For this review, use the dimensioned drawing (mm, ordinates from the lowest corner) and the shaded views. Round coordinates to 2 decimals unless told otherwise and drop trailing zeros. Write each loop counter-clockwise with the first axis right and the second up, starting at its lowest first coordinate (ties: lowest second). Pieces come first, ordered by that corner, then holes. Notation, with made-up numbers: M -28,81 L -7,81 A31 ccw -7,119 Z; hole C 64.5,-10.75 d8. An arc over 180 degrees is marked long. Answer in a Markdown table with one row per item.
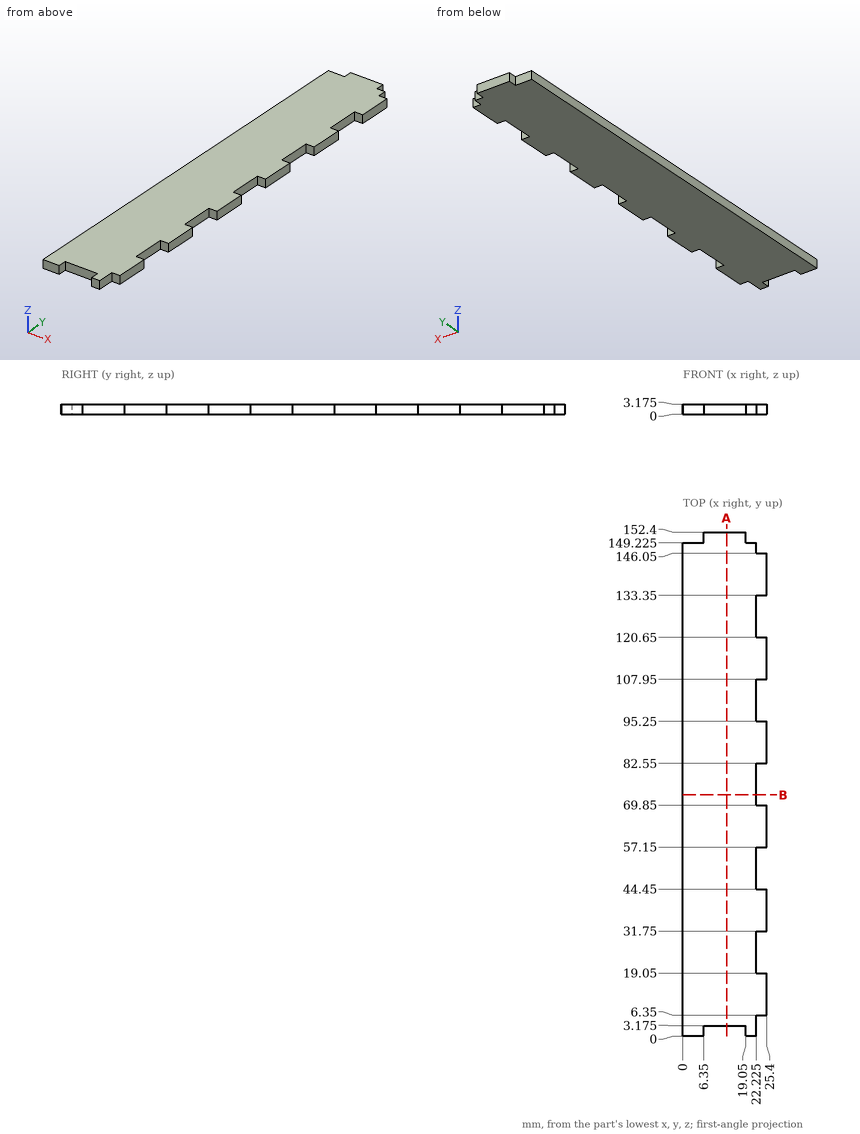
Q1. Take a section at B-B (y = 73). State the section outline as (x, z) points (3 decimals).
Found:
| item | result |
|---|---|
| outline | M 0,0 L 22.225,0 L 22.225,3.175 L 0,3.175 Z |
Q2. Insertion check: P1, Ø1.6, axis at x = 23.5, z = 1.5, coming from the -Y side; P2, Ø1, axis at x = 23.5, z = 1.5, coming from the +Y side; P3, Ø1.6, axis at y = 53, z = 1.5, coming from the +X side (3 decimals). Each pin has a flat end and moves straight along its axis. Give the tip position at first contact, or say it passes through.
Found:
| item | result |
|---|---|
| P1 | y = 6.35 |
| P2 | y = 146.05 |
| P3 | x = 22.225 |
Q3. For probe 1 along Y at (x, z) = (24.25, 2.6); probe 2 along X at (y, z) = (79.5, 2.1) (3 decimals); probe 3 along Y at (x, z) = (7.75, 0.4) (3 decimals), list the stretches that pass through material, from the lowest coordinate up.
Found:
| item | result |
|---|---|
| probe 1 | 6.35 to 19.05, 31.75 to 44.45, 57.15 to 69.85, 82.55 to 95.25, 107.95 to 120.65, 133.35 to 146.05 |
| probe 2 | 0 to 22.225 |
| probe 3 | 3.175 to 152.4 |
Q4. Take a section at A-A (x = 13.25). State the section outline as (y, z) points (3 decimals).
Found:
| item | result |
|---|---|
| outline | M 3.175,0 L 152.4,0 L 152.4,3.175 L 3.175,3.175 Z |
